Read the model definition and answer for the solid it produces. Units are mm, in the model's axes. A direction names the side the tool comes from. Round coordinates to 2 decimals unless told otherwise and drop trailing zeros. Loops run counter-clockwise (first coordinate to the right, second up) from the corner with the lowest first, then second, coordinate; pieces in that order, holes last. Notation, with made-up numbers: M -25.5,-2 L -1.5,-2 A21 cw -1.5,2 Z; hole C 41,47.25 d3. An arc over 180 degrees is marked long. Write each question's results on one line, items separated by ' | '.
```python
from build123d import *

# Parameters (mm, degrees)
SKETCH1_R           = 2.1
SKETCH1_R_2         = 7
BOSS_EXTRUDE1_DEPTH = 4
FILLET1_R           = 2
SKETCH2_R           = 3.9
CUT_EXTRUDE1_DEPTH  = 2.4


with BuildPart() as part:
    # Sketch1 → Boss-Extrude1 (new body)
    with BuildSketch(Plane(origin=(0, 0, 0), x_dir=(1, 0, 0), z_dir=(0, 1, 0))):
        with BuildLine():
            ThreePointArc((-20.156225815, 0), (0, 20.156225815), (20.156225815, 0))
            ThreePointArc((20.156225815, 0), (25.4, -5.243774185), (30.643774185, 0))
            add(Edge.make_bspline(
                [(-46.474516908, 36.934762739), (-23.164206568, 39.351897946), (33.373901801, 38.120150773), (30.643774185, 0)],
                knots=[0, 0, 0, 0, 1, 1, 1, 1], degree=3))
            ThreePointArc((-46.474516908, 36.934762739), (-59.166363236, 25.114100216), (-48.276532762, 11.615114404))
            add(Edge.make_bspline(
                [(-48.276532762, 11.615114404), (-40.793059369, 8.635332343), (-34.627763453, 3.802891886), (-29.780645012, -2.882206965)],
                knots=[0.158174001, 0.158174001, 0.158174001, 0.158174001, 0.985694322, 0.985694322, 0.985694322, 0.985694322], degree=3))
            add(Edge.make_bspline(
                [(-29.780645012, -2.882206965), (-29.696850917, -2.997774969), (-29.613450765, -3.113896649), (-29.530444557, -3.230572003)],
                knots=[0.985694322, 0.985694322, 0.985694322, 0.985694322, 1, 1, 1, 1], degree=3))
            ThreePointArc((-29.530444557, -3.230572003), (-23.691484685, -4.957634831), (-20.156225815, 0))
        make_face()
        with Locations(Location((-25.4, 0, 0), (0, 0, 270))):
            Circle(SKETCH1_R, mode=Mode.SUBTRACT)
        with Locations(Location((25.4, 0, 0), (0, 0, 270))):
            Circle(SKETCH1_R, mode=Mode.SUBTRACT)
        with Locations(Location((-46.474516908, 24.210813251, 0), (0, 0, 270))):
            Circle(SKETCH1_R_2, mode=Mode.SUBTRACT)
        with BuildLine():
            Line((-30.18742995, 5.773258566), (-35.582829026, 12.279679392))
            add(Edge.make_bspline(
                [(-34.116347467, 20.501234406), (-35.438334408, 17.651696826), (-35.927161595, 14.911178488), (-35.582829026, 12.279679392)],
                knots=[0, 0, 0, 0, 0.482948313, 0.482948313, 0.482948313, 0.482948313], degree=3))
            ThreePointArc((-34.116347467, 20.501234406), (-29.755996604, 21.898993805), (-27.020904781, 25.57127698))
            add(Edge.make_bspline(
                [(-27.020904781, 25.57127698), (-17.402553682, 30.495527598), (-7.5, 25.57127698)],
                knots=[0, 0, 0, 1, 1, 1], degree=2))
            add(Edge.make_bspline(
                [(-7.5, 25.57127698), (-21.293728183, 21.457376491), (-25.4, 7.5)],
                knots=[0, 0, 0, 1, 1, 1], degree=2))
            ThreePointArc((-25.4, 7.5), (-27.944657222, 7.0551201), (-30.18742995, 5.773258566))
        make_face(mode=Mode.SUBTRACT)
        with Locations(Location((-34.116347467, 28.001234406, 0), (0, 0, 270))):
            Circle(SKETCH1_R, mode=Mode.SUBTRACT)
        with Locations(Location((0, 25.57127698, 0), (0, 0, 270))):
            Circle(SKETCH1_R, mode=Mode.SUBTRACT)
    extrude(amount=BOSS_EXTRUDE1_DEPTH)

    # Fillet1
    fillet1_edges = [part.edges().sort_by_distance(p)[0] for p in [
        (-34.116347467, 2, -20.501234406),
        (-35.582829026, 2, -12.279679392),
        (-30.18742995, 2, -5.773258566),
        (-25.4, 2, -7.5),
        (-7.5, 2, -25.57127698),
        (-27.020904781, 2, -25.57127698),
    ]]
    fillet(fillet1_edges, radius=FILLET1_R)

    # Sketch2 → Cut-Extrude1 (cut)
    with BuildSketch(Plane(origin=(0, 4, 0), x_dir=(1, 0, 0), z_dir=(0, 1, 0))):
        with Locations(Location((-34.116347467, 28.001234406, 0), (0, 0, 270))):
            Circle(SKETCH2_R)
        with Locations(Location((0, 25.57127698, 0), (0, 0, 270))):
            Circle(SKETCH2_R)
        with Locations(Location((-25.4, 0, 0), (0, 0, 270))):
            Circle(SKETCH2_R)
        with Locations(Location((25.4, 0, 0), (0, 0, 270))):
            Circle(SKETCH2_R)
    extrude(amount=-CUT_EXTRUDE1_DEPTH, mode=Mode.SUBTRACT)


solid = part.part
```
1. Determine the mould class of faces 1 (the face through (-13, 4, -20)), 2 (the face through (-0.44, 1.97, -20.15)), 3 (the face through (-59.145, 1.972, -25.38)), 4 (the face through (-27, 1.6, 2)) for opening direction Z: released by +Z, released by -Z, zero draft, split by the parting line, or undercut.
Completed:
face 1: zero draft | face 2: released by +Z | face 3: split by the parting line | face 4: undercut
2. Which of the six approach directions +Z, -Z, +X, -X, +Y, -Y give full straight-line access (tool end or side, diameter ignored) to faces 5 (the face through (25.285, 1.972, 5.243)), 6 (the face through (-22.112, 2.817, 2.097)), 7 (the face through (-27.74, 1.972, -7.125))?
Completed:
face 5: +Z, +Y, -Y | face 6: +Y | face 7: +Y, -Y
3. Find section B-B, the plane z = 1. Count the separate pieces of the cut face and the enclosed holes in it, then the cut area to 3 significant figures.
Completed:
separate pieces: 4 | enclosed holes: 0 | area: 37.0 mm2
4. Given P1, Ø1.5, axis at x = -12.5, y = 3, coming from the +Z side; P2, Ø6.5, axis at x = -34.12, z = -28, coming from the +Y side; P3, Ø1.5, axis at y = 2, z = -9, coming from the -X side, each flat-ended and moving along its own axis, determine where each tip first touches the part or whether it passes through.
Completed:
P1: stops at z = -15.19 | P2: stops at y = 1.6 | P3: stops at x = -44.22
5. Find section A-A, the plane x = -51.5. Give the vertices of the cut face in (y, z), then the cut area to 3 significant figures.
Completed:
outline: M 0,-35.9 L 4,-35.9 L 4,-29.08 L 0,-29.08 Z; M 0,-19.34 L 4,-19.34 L 4,-12.52 L 0,-12.52 Z | area: 54.5 mm2
6. Find the intervals of material crossed by L1, parallel to X at y = 3.4, z = 0.5; L2, parallel to X at y = 1.4, z = -21.5; L3, parallel to X at y = 3.6, z = -0.5, in increasing order.
Completed:
L1: x = -31.63 to -29.27, -21.53 to -20.18, 20.18 to 21.53, 29.27 to 30.62 | L2: x = -58.91 to -52.93, -40.02 to -30.38, -15.95 to 23.68 | L3: x = -32.48 to -29.27, -21.53 to -20.15, 20.15 to 21.53, 29.27 to 30.68
